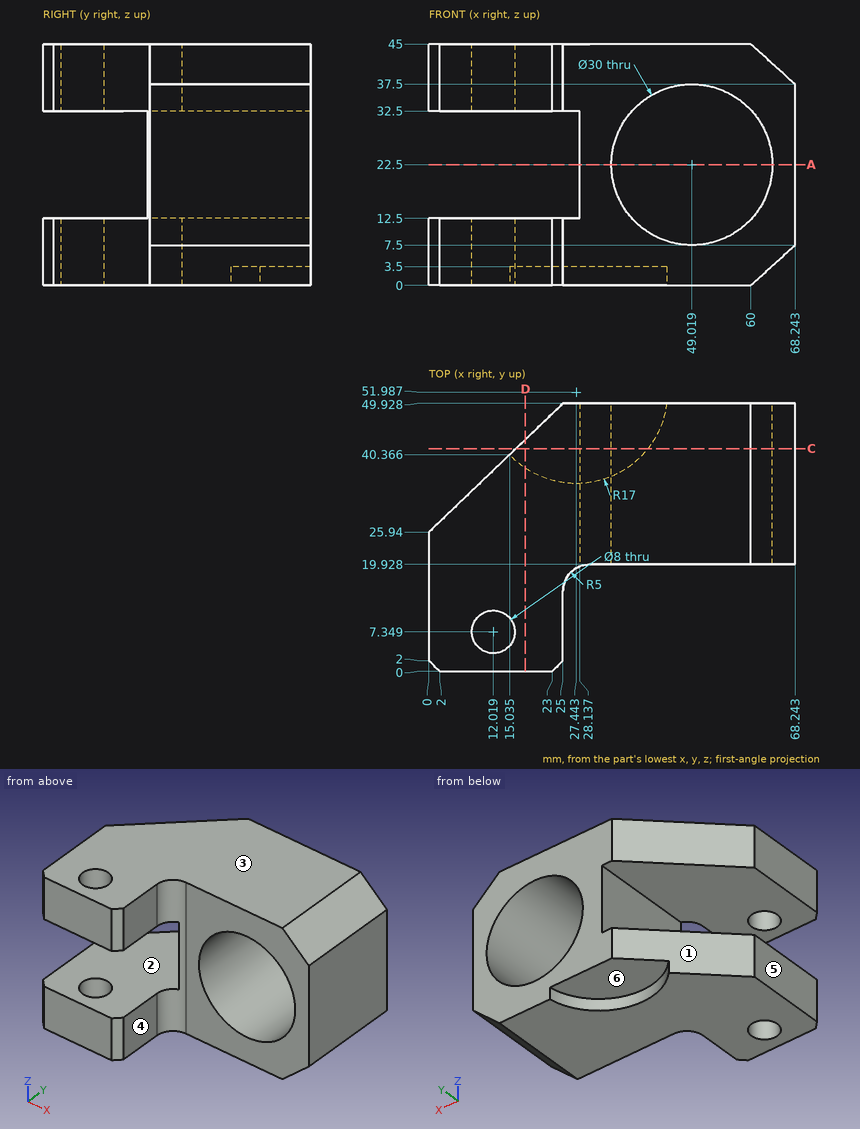
Check sheet for the drawn part. Datum: minimum x, y, z corner. Units: mm. A direction names the side the tool comes from. Round coordinates to 2 decimals unless told otherwise and drop trailing zeros. Loops run counter-clockwise (first coordinate to the right, second up) from the corner with the lowest first, then second, coordinate; pieces in that order, holes last. Notation, with made-up numbers: (30.25, -8) - (49.25, -8) arc R24 cw to (49.25, 4) - close; hole circle Ø10 at (-1, 5.25). An arc over 180 degrees is marked (long way). Answer as a JSON object with one key per item and string values. Group by question number.
Q1. Sectioned sample at C-C, the plane y = 41.5. Enter the section's corners in (x, z), plus the area to 3 significant figures.
Q2. Sectioned sample at A-A, the plane z = 22.5. Enter the section's corners in (x, y).
Q3. Scan lines: line 1 along Z through (x, y) = (18.5, 43); line 2 along Z through (x, y) = (15, 20); line 3 along X through (y, z) = (30, 22.5). Record each from-to range of solid material in increasing order. Write a range as [from, to].
Q4. Gauge pin test, flat ends, axial feed: P1, Ø6, axis at y = 37.5, z = 26, coming from the -X side; P2, Ø14, axis at y = 5.5, z = 4, coming from the +X side; P3, Ø5, axis at y = 16.5, z = 24, coming from the +X side; P4, Ø4, axis at x = 35, y = 43.5, coming from the -Z side. Record the tip position at first contact, or that the pin passes through.
Q5. Set-up check for the marked faces 4, 5 and 6: record each of +Z, -Z, +X, -X, +Y, -Y from which the full face is reachable in a straight line by a thin tool's end or side.
Q6. Mould release check, pull along Z, two halves, no side actions. Record for the marked faces 1, 2 and 3: released by +Z, released by -Z, zero draft, split by the parting line, or undercut.
Q7. Sectioned sample at D-D, the plane x = 18. Enter the section's corners in (y, z), plus the area to 3 significant figures.
Solution:
{
 "1": {"outline": "(16.22, 3.5) - (40.82, 3.5) - (40.82, 0) - (60, 0) - (68.24, 7.5) - (68.24, 37.5) - (60, 45) - (16.22, 45) - (16.22, 32.5) - (28.14, 32.5) - (28.14, 12.5) - (16.22, 12.5) - close; hole circle Ø30 at (49.02, 22.5)", "area": "1,250 mm²"},
 "2": {"outline": "(28.14, 19.57) arc R5 cw to (30, 19.93) - (34.02, 19.93) - (34.02, 49.93) - (28.14, 49.93) - close; (64.02, 19.93) - (68.24, 19.93) - (68.24, 49.93) - (64.02, 49.93) - close"},
 "3": {"line 1": "z = [3.5, 12.5], [32.5, 45]", "line 2": "z = [0, 12.5], [32.5, 45]", "line 3": "x = [28.14, 34.02], [64.02, 68.24]"},
 "4": {"P1": "stops at x = 28.14", "P2": "stops at x = 25", "P3": "passes through", "P4": "stops at z = 3.5"},
 "5": {"face 4": "+Z, -Z, +X, -Y", "face 5": "+Z, -Z, -X, +Y, -Y", "face 6": "-Z, +Y"},
 "6": {"face 1": "zero draft", "face 2": "undercut", "face 3": "released by +Z"},
 "7": {"outline": "(0, 0) - (37.85, 0) - (37.85, 3.5) - (43.21, 3.5) - (43.21, 12.5) - (0, 12.5) - close; (0, 32.5) - (43.21, 32.5) - (43.21, 45) - (0, 45) - close", "area": "1,060 mm²"}
}
